Read the model definition and answer for the solid it produces. Units are mm, in the model's axes. A direction names the side the tool comes from. Coordinates: 2 decimals unless noted, no trailing zeros. Loops run counter-clockwise (first coordinate to the right, second up) from the corner with the lowest first, then second, coordinate; pieces in that order, holes last. Notation, with made-up numbers: (76, 41.5) - (106, 41.5) arc R8 cw to (106, 46.5) - close; hole circle Ø7 at (61, 3.25). An arc over 180 degrees is marked (long way). One line per item, written item: value. Start each with the question number.
from build123d import *

# Parameters (mm, degrees)
SKETCH_1_R          = 6
EXTRUDE_1_DEPTH     = 6
CUT_EXTRUDE_1_DEPTH = 10
EXTRUDE_START       = -6
SKETCH_3_R          = 2.5
EXTRUDE_2_DEPTH     = 6
FILLET_2_R          = 5


with BuildPart() as part:
    # 草图1 → 凸台-拉伸1 (new body)
    with BuildSketch(Plane(origin=(0, 0, 0), x_dir=(0, 0, -1), z_dir=(1, 0, 0))):
        with BuildLine():
            Line((15, 0), (17.5, -200))
            ThreePointArc((17.5, -200), (0, -217.5), (-17.5, -200))
            Line((-17.5, -200), (-15, 0))
            ThreePointArc((-15, 0), (0, 15), (15, 0))
        make_face()
        Circle(SKETCH_1_R, mode=Mode.SUBTRACT)
        with Locations((0, -200)):
            Circle(SKETCH_1_R, mode=Mode.SUBTRACT)
    extrude(amount=EXTRUDE_1_DEPTH)

    # 草图2 → 切除-拉伸1 (cut)
    with BuildSketch(Plane(origin=(6, 0, 0), x_dir=(0, 0, -1), z_dir=(1, 0, 0))):
        with BuildLine():
            Line((5, -25), (5, -85))
            ThreePointArc((5, -85), (0, -90), (-5, -85))
            Line((-5, -85), (-5, -25))
            ThreePointArc((-5, -25), (0, -20), (5, -25))
        make_face()
        with BuildLine():
            Line((4.5, -105), (4.5, -160))
            ThreePointArc((4.5, -160), (0, -164.5), (-4.5, -160))
            Line((-4.5, -160), (-4.5, -105))
            ThreePointArc((-4.5, -105), (0, -100.5), (4.5, -105))
        make_face()
    extrude(amount=-CUT_EXTRUDE_1_DEPTH, mode=Mode.SUBTRACT)

    # 草图3 → 凸台-拉伸2 (add)
    with BuildSketch(Plane(origin=(6, 0, 0), x_dir=(0, 0, -1), z_dir=(1, 0, 0)).offset(EXTRUDE_START)):
        with BuildLine():
            Line((-15.155444566, -208.75), (-0.155444566, -234.730762114))
            ThreePointArc((-0.155444566, -234.730762114), (23.75, -241.13620668), (30.155444566, -217.230762114))
            Line((30.155444566, -217.230762114), (17.440089003, -195.207120242))
            Line((17.440089003, -195.207120242), (17.494532104, -199.562568349))
            ThreePointArc((17.494532104, -199.562568349), (15.263627142, -208.559888228), (8.75, -215.155444566))
            ThreePointArc((8.75, -215.155444566), (-4.529333289, -216.90370196), (-15.155444566, -208.75))
        make_face()
        with Locations((15, -225.980762114)):
            Circle(SKETCH_3_R, mode=Mode.SUBTRACT)
    extrude(amount=EXTRUDE_2_DEPTH)

    # 圆角2
    fillet_2_edges = [part.edges().sort_by_distance(p)[0] for p in [
        (3, -195.207120242, -17.440089003),
    ]]
    fillet(fillet_2_edges, radius=FILLET_2_R)


solid = part.part
1) For faces 5 (the cylindrical face through (3, -100.5, 0.1)), 6 (the flat face through (0, -141, -7)), determine the directions among +Z, -Z, +X, -X, +Y, -Y from which every point of the face is accessible in a straight line to the end or side of a thin tool.
2) Flat-ended cylindrical pins translate along their axes: P1, Ø1.8, axis at x = 1.5, y = -126.5, coming from the -Z side; P2, Ø7, axis at y = -200, z = 0, coming from the -X side; P3, Ø1.8, axis at x = 3, y = -45.5, coming from the +Z side; P4, Ø3, axis at x = 3, y = -45, coming from the -Z side. Find the tip coordinate at first contact, or state that the pin passes through.
3) Section C-C, the plane z = 12 is taken. Determine the outline of the cut face in (x, y).
4) Section A-A, the plane y = -42.5 is taken. Determine the outline of the cut face in (x, z).
5) Section D-D, the plane y = -157.5 is taken. Determine the outline of the cut face in (x, z), and give its area (3 significant figures).
6) Straight lines are drawn through the part: L1, parallel to Y at x = 0.6, z = -1; L2, parallel to Z at x = 2.2, y = -51; L3, parallel to Y at x = 3.45, z = -3. For each, find the intervals that lie inside material, in ascending order.
7) Determine the mould class of faces 1 (the cylindrical face through (3, 15, 0)), 2 (the cylindrical face through (2.958, -204.591, 16.887)), 3 (the cylindrical face through (3, 0, 6)), 4 (the flat face through (6, -141, -7)) for opening direction Z: released by +Z, released by -Z, zero draft, split by the parting line, or undercut.
Answer below:
1. face 5: +X, -X
1. face 6: +Z, -Z, -X, +Y, -Y
2. P1: z = -16.59
2. P2: through
2. P3: z = 15.58
2. P4: z = -15.58
3. outline: (0, -214.22) - (6, -214.22) - (6, 9) - (0, 9) - close
4. outline: (0, -15.53) - (6, -15.53) - (6, -5) - (0, -5) - close; (0, 5) - (6, 5) - (6, 15.53) - (0, 15.53) - close
5. outline: (0, -16.97) - (6, -16.97) - (6, -4.5) - (0, -4.5) - close; (0, 4.5) - (6, 4.5) - (6, 16.97) - (0, 16.97) - close
5. area: 150 mm2
6. L1: -236.48 to -205.92, -194.08 to -164.39, -100.61 to -89.9, -20.1 to -5.92, 5.92 to 14.97
6. L2: -15.64 to -5, 5 to 15.64
6. L3: -238.72 to -205.2, -194.8 to -163.35, -101.65 to -89, -21 to -5.2, 5.2 to 14.7
7. face 1: split by the parting line
7. face 2: released by +Z
7. face 3: undercut
7. face 4: zero draft
